Could you check a few things on this model? Use its own coordinates, in mm. A direction names the side the tool comes from. Coordinates: 2 decimals unless noted, no trailing zeros. Write each loop counter-clockwise with the first axis right and the second up, starting at its lowest first coordinate (ties: lowest second). Pieces come first, ordered by that corner, then holes.
Item 1: For P1, Ø14.5, axis at x = -19, z = 7.5, coming from the +Y side; P2, Ø3, axis at x = -18.5, z = 11.5, coming from the +Y side; P3, Ø7, axis at x = -21, z = 9.5, coming from the +Y side, each with a flat end and sliding along its axis, tell me the tip position at first contact or that it passes through.
Item 2: If I drill on probe 1 along Y at (x, z) = (-23.5, 8); probe 2 along Y at (x, z) = (-11.5, 11.5); probe 3 along Z at (x, y) = (-18.5, 38), over which ranges is the centre line in solid material (lowest first)?
Item 3: Which directions (+Z, -Z, +X, -X, +Y, -Y) give clear straight access to the entire face, cutting with the end or side of a thin tool? Please do faces 1 (the flat face through (-22, -25, 15)), 2 (the flat face through (0, 0, 2)), 3 (the flat face through (-16, 0, 11)), 4 (the flat face through (-20, -22, 10)), 5 (the flat face through (-27.5, -2, 11)).
Item 4: I want a section at B-B on z = 13.5. Please give me the cut outline in (x, y).
Item 5: I want a section at D-D on y = -15. Please give me the cut outline in (x, z), then the cut area to 3 significant figures.
Item 6: I want a section at A-A on x = -23. State how many separate pieces and enclosed holes the cut face has, then the cut area to 3 significant figures.
Item 7: Thinking about a two-plate mould opening in Z: for faces 6 (the flat face through (-11, 19, 0)), 7 (the flat face through (5, 35, 3)), 8 (the flat face through (-25, -12, 15)), 9 (the flat face through (-22, -26, 10)), which applies, +Z half, -Z half, draft (parallel to the pull), parting line (faces both ways), or undercut?
from build123d import *

# Parameters (mm, degrees)
F1_W      = 0.5
F1_H      = 7.5
F1_H_2    = 1
F2_DEPTH  = 11
F1_W_2    = 25
F1_H_3    = 2
F3_DEPTH  = 2.5
F6_DEPTH  = 1
F1_W_3    = 70
F1_H_4    = 5
F7_DEPTH  = 23
F9_W      = 70
F9_H      = 5
F10_DEPTH = 12.5
F11_SIZE  = 4.99999
F13_R     = 2


# Not quite as in the source:
# - a fillet or chamfer is up to 0.001 mm smaller than in the source, because OpenCascade refuses the exact size


with BuildPart() as f2:
    # F1 (on offset) → F2 (new body)
    with BuildSketch(Plane.YZ.offset(-27.5)):
        Polygon((-26, 6), (-26, 15), (-27, 15), (-27, 5), (-22, 5), (-22, 7.5), (-22.5, 7.5), (-22.5, 15), (-23, 15), (-23, 6), align=None)
        Polygon((-27, 15), (-26, 15), (-23, 15), (-22.5, 15), (-22.5, 16), (-27, 16), align=None)
        with Locations((-22.25, 11.25)):
            Rectangle(F1_W, F1_H)
        with Locations((-22.25, 15.5)):
            Rectangle(F1_W, F1_H_2)
    extrude(amount=F2_DEPTH)

    # F1 (on offset) → F3 (join)
    with BuildSketch(Plane.YZ.offset(-27.5)):
        with BuildLine():
            Line((-27.5, 2), (-2.5, 2))
            Line((-2.5, 2), (-2.5, 15))
            ThreePointArc((-2.5, 15), (-15, 27.5), (-27.5, 15))
            Line((-27.5, 15), (-27.5, 2))
        make_face()
        Polygon((-27, 5), (-27, 15), (-27, 16), (-22.5, 16), (-22.5, 22.5), (-7.5, 22.5), (-7.5, 7.5), (-22, 7.5), (-22, 5), align=None, mode=Mode.SUBTRACT)
        Polygon((-22, 16), (-22, 15), (-22, 7.5), (-7.5, 7.5), (-7.5, 22.5), (-22.5, 22.5), (-22.5, 16), align=None)
        with Locations((-15, 1)):
            Rectangle(F1_W_2, F1_H_3)
    extrude(amount=F3_DEPTH)

    # F5 (on offset) → F6 (join)
    with BuildSketch(Plane.YZ.offset(-16.5)):
        Polygon((-26, 14), (-26, 15), (-23, 15), (-23, 13.8), (-22, 16), (-27, 16), (-27, 5), (-26, 7.2), align=None)
        Polygon((-26, 6), (-26, 7.2), (-27, 5), (-25, 5), (-24, 5), (-22, 5), (-22, 16), (-23, 13.8), (-23, 6), align=None)
        Polygon((-23, 15), (-26, 15), (-26, 14), (-26, 7.2), (-25, 9.4), (-25, 14.75), (-24, 14.75), (-24, 11.6), (-23, 13.8), align=None)
        Polygon((-25, 9.4), (-26, 7.2), (-26, 6), (-23, 6), (-23, 13.8), (-24, 11.6), (-24, 6.25), (-25, 6.25), align=None)
    extrude(amount=F6_DEPTH)

    # F1 (on offset) → F7 (join)
    with BuildSketch(Plane.YZ.offset(-27.5)):
        with BuildLine():
            Line((-2.5, 0), (0, 0))
            Line((0, 0), (0, 5))
            Line((0, 5), (0, 15))
            ThreePointArc((0, 15), (-15, 30), (-30, 15))
            Line((-30, 15), (-30, 0))
            Line((-30, 0), (-27.5, 0))
            Line((-27.5, 0), (-27.5, 2))
            Line((-27.5, 2), (-27.5, 15))
            ThreePointArc((-27.5, 15), (-15, 27.5), (-2.5, 15))
            Line((-2.5, 15), (-2.5, 2))
            Line((-2.5, 2), (-2.5, 0))
        make_face()
        with Locations((35, 2.5)):
            Rectangle(F1_W_3, F1_H_4)
        with Locations((-15, 1)):
            Rectangle(F1_W_2, F1_H_3)
    extrude(amount=F7_DEPTH)

    # F9 (on offset) → F10 (join)
    with BuildSketch(Plane.YZ.offset(-7.5)):
        with Locations((35, 2.5)):
            Rectangle(F9_W, F9_H)
    extrude(amount=F10_DEPTH)

    # F11 (size 5 in the source; OpenCascade refuses exactly that, so slightly less here)
    f11_edges = [f2.edges().sort_by_distance(p)[0] for p in [
        (-11.25, 70, 5),
    ]]
    chamfer(f11_edges, length=F11_SIZE)

    # F13
    f13_edges = [f2.edges().sort_by_distance(p)[0] for p in [
        (-16, 0, 5),
    ]]
    fillet(f13_edges, radius=F13_R)


solid = f2.part
Response values:
1. P1: stops at y = 69.75
1. P2: stops at y = 0
1. P3: stops at y = 0.27
2. probe 1: y = -30 to -27.5, -27 to -26, -23 to -22, -2.5 to 0
2. probe 2: y = -30 to -27.5, -2.5 to 0
2. probe 3: z = 0 to 5
3. face 1: -X
3. face 2: +Z, -Z, +X, -Y
3. face 3: +Z, +X, -X, +Y
3. face 4: +X
3. face 5: +Z, -Z, -X, +Y, -Y
4. outline: (-27.5, -30) - (-4.5, -30) - (-4.5, -27.5) - (-25, -27.5) - (-25, -27) - (-15.5, -27) - (-15.5, -25) - (-16.5, -25) - (-16.5, -26) - (-27.5, -26) - close; (-27.5, -23) - (-16.5, -23) - (-16.5, -24) - (-15.5, -24) - (-15.5, -22) - (-25, -22) - (-25, -2.5) - (-4.5, -2.5) - (-4.5, 0) - (-27.5, 0) - close
5. outline: (-27.5, 0) - (-4.5, 0) - (-4.5, 2) - (-25, 2) - (-25, 27.5) - (-4.5, 27.5) - (-4.5, 30) - (-27.5, 30) - close
5. area: 167 mm2
6. separate pieces: 2
6. enclosed holes: 2
6. area: 599 mm2
7. face 6: -Z half
7. face 7: draft
7. face 8: undercut
7. face 9: undercut
